Geometry check sheet. Reference: the model listing, model coordinates, mm. Face numbers are marked on the shaded views. Round coordinates to 2 decimals unless told otherwise and drop trailing zeros. Write each loop counter-clockwise with the first axis right and the second up, starting at its lowest first coordinate (ties: lowest second). Pieces come first, ordered by that corner, then holes. Notation, with made-up numbers: (-0.5, -22.5) - (47.5, -22.5) arc R18 ccw to (47.5, -11.5) - close; hole circle Ø11 at (6, 49.5). An arc over 180 degrees is marked (long way). Return JSON: item names as keys, results as strings. Group by question number.
from build123d import *

# Parameters (mm, degrees)
SKETCH2_R           = 21
BOSS_EXTRUDE1_DEPTH = 10
CUT_EXTRUDE1_REACH  = 77.44
SKETCH3_R           = 1.75
SKETCH5_W           = 4
SKETCH5_H           = 1


with BuildPart() as part:
    # Sketch2 → Boss-Extrude1 (new body)
    # profile 1 of 6: a face of its own
    with BuildSketch(Plane(origin=(0, 0, 0), x_dir=(1, 0, 0), z_dir=(0, 1, 0))):
        with BuildLine():
            ThreePointArc((-39.742001703, 30.095205518), (-35.527778851, 29.794741171), (-31.819805153, 31.819805153))
            Line((-31.819805153, 31.819805153), (-42.426406871, 42.426406871))
            ThreePointArc((-42.426406871, 42.426406871), (-44.451470854, 35.527778851), (-39.742001703, 30.095205518))
        make_face()
    # profile 2 of 6: a face of its own
    with BuildSketch(Plane(origin=(0, 0, 0), x_dir=(1, 0, 0), z_dir=(0, 1, 0))):
        with BuildLine():
            Line((-42.426406871, 42.426406871), (-31.819805153, 31.819805153))
            ThreePointArc((-31.819805153, 31.819805153), (0, 45), (31.819805153, 31.819805153))
            ThreePointArc((31.819805153, 31.819805153), (35.527778851, 29.794741171), (39.742001703, 30.095205518))
            ThreePointArc((39.742001703, 30.095205518), (44.451470854, 35.527778851), (42.426406871, 42.426406871))
            ThreePointArc((42.426406871, 42.426406871), (0, 60), (-42.426406871, 42.426406871))
        make_face()
    # profile 3 of 6: a face of its own
    with BuildSketch(Plane(origin=(0, 0, 0), x_dir=(1, 0, 0), z_dir=(0, 1, 0))):
        with BuildLine():
            ThreePointArc((31.819805153, 31.819805153), (0, 45), (-31.819805153, 31.819805153))
            ThreePointArc((-31.819805153, 31.819805153), (-33.665365801, 29.860394262), (-35.390472848, 27.794143836))
            add(Edge.make_bspline(
                [(-35.390472848, 27.794143836), (-32.245912853, 25.570807212), (-24.806129807, 15.839794796), (-24.750821328, 4.074395815), (-23.058627279, -4.533178579)],
                knots=[0.115209689, 0.115209689, 0.115209689, 0.115209689, 0.392292763, 1, 1, 1, 1], degree=3))
            ThreePointArc((-23.058627279, -4.533178579), (-2.277307506, 23.38939654), (23.5, 0))
            ThreePointArc((23.5, 0), (23.38939654, -2.277307506), (23.058627279, -4.533178579))
            add(Edge.make_bspline(
                [(35.390472848, 27.794143836), (32.245912853, 25.570807212), (24.806129807, 15.839794796), (24.750821328, 4.074395815), (23.058627279, -4.533178579)],
                knots=[0.115209689, 0.115209689, 0.115209689, 0.115209689, 0.392292763, 1, 1, 1, 1], degree=3))
            ThreePointArc((35.390472848, 27.794143836), (33.665365801, 29.860394262), (31.819805153, 31.819805153))
        make_face()
    # profile 4 of 6: a face of its own
    with BuildSketch(Plane(origin=(0, 0, 0), x_dir=(1, 0, 0), z_dir=(0, 1, 0))):
        with BuildLine():
            ThreePointArc((-35.390472848, 27.794143836), (-33.665365801, 29.860394262), (-31.819805153, 31.819805153))
            ThreePointArc((-31.819805153, 31.819805153), (-35.527778851, 29.794741171), (-39.742001703, 30.095205518))
            add(Edge.make_bspline(
                [(-39.742001703, 30.095205518), (-38.146305527, 29.500581015), (-36.697964408, 28.718595549), (-35.390472848, 27.794143836)],
                knots=[0, 0, 0, 0, 0.115209689, 0.115209689, 0.115209689, 0.115209689], degree=3))
        make_face()
    # profile 5 of 6: a face of its own
    with BuildSketch(Plane(origin=(0, 0, 0), x_dir=(1, 0, 0), z_dir=(0, 1, 0))):
        with BuildLine():
            ThreePointArc((39.742001703, 30.095205518), (35.527778851, 29.794741171), (31.819805153, 31.819805153))
            ThreePointArc((31.819805153, 31.819805153), (33.665365801, 29.860394262), (35.390472848, 27.794143836))
            add(Edge.make_bspline(
                [(39.742001703, 30.095205518), (38.146305527, 29.500581015), (36.697964408, 28.718595549), (35.390472848, 27.794143836)],
                knots=[0, 0, 0, 0, 0.115209689, 0.115209689, 0.115209689, 0.115209689], degree=3))
        make_face()
    # profile 6 of 6: a face of its own
    with BuildSketch(Plane(origin=(0, 0, 0), x_dir=(1, 0, 0), z_dir=(0, 1, 0))):
        with BuildLine():
            ThreePointArc((23.5, 0), (-2.277307506, 23.38939654), (-23.058627279, -4.533178579))
            ThreePointArc((-23.058627279, -4.533178579), (0, -23.5), (23.058627279, -4.533178579))
            ThreePointArc((23.058627279, -4.533178579), (23.38939654, -2.277307506), (23.5, 0))
        make_face()
        with Locations(Location((0, 0, 0), (0, 0, 270))):
            Circle(SKETCH2_R, mode=Mode.SUBTRACT)
    extrude(amount=BOSS_EXTRUDE1_DEPTH)

    # Sketch3 → Cut-Extrude1 (cut, up to next)
    with BuildSketch(Plane(origin=(0, 10, 0), x_dir=(1, 0, 0), z_dir=(0, 1, 0)), mode=Mode.PRIVATE) as cut_extrude1_sk1:
        with Locations(Location((-37.123106012, 37.123106012, 0), (0, 0, 270))):
            Circle(SKETCH3_R)
    cut_extrude1_tool1 = extrude(cut_extrude1_sk1.sketch, amount=-CUT_EXTRUDE1_REACH, mode=Mode.PRIVATE) & part.part
    # Sketch3 → Cut-Extrude1 (cut, up to next)
    with BuildSketch(Plane(origin=(0, 10, 0), x_dir=(1, 0, 0), z_dir=(0, 1, 0)), mode=Mode.PRIVATE) as cut_extrude1_sk2:
        with Locations(Location((37.123106012, 37.123106012, 0), (0, 0, 270))):
            Circle(SKETCH3_R)
    cut_extrude1_tool2 = extrude(cut_extrude1_sk2.sketch, amount=-CUT_EXTRUDE1_REACH, mode=Mode.PRIVATE) & part.part
    add(cut_extrude1_tool1.solids().sort_by_distance((-37.123106, 10, -37.123106))[0], mode=Mode.SUBTRACT)
    add(cut_extrude1_tool2.solids().sort_by_distance((37.123106, 10, -37.123106))[0], mode=Mode.SUBTRACT)

    # Sketch5 → Revolve1 (revolve)
    with BuildSketch(Plane.XY, mode=Mode.PRIVATE) as revolve1_sk:
        with Locations((-21.058627279, 7.5)):
            Rectangle(SKETCH5_W, SKETCH5_H)
    revolve(revolve1_sk.sketch.rotate(Axis((0, 10, 0), (0, -1, 0)), 270), axis=Axis((0, 10, 0), (0, -1, 0)))


solid = part.part
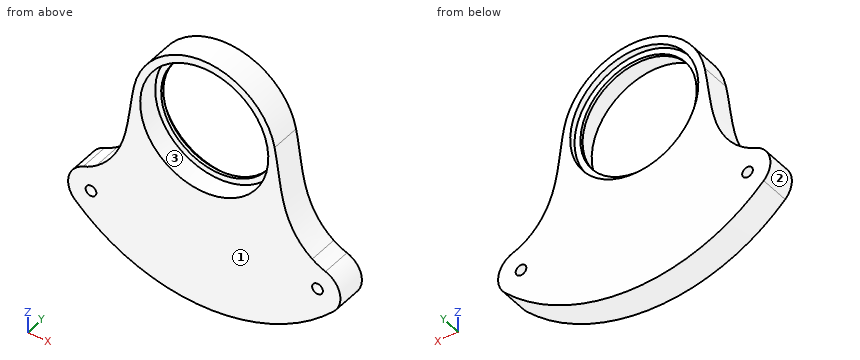
1. Material ranges on line 1 along X through (y, z) = (1.75, -38); line 2 along Z through (x, y) = (0, 9.5); line 3 along Z through (x, y) = (11, 1.75), recorded low to high.
2. Mould release check, pull along Z, two halves, no side actions. Record for the marked faces 1, 2 and 3: pulls with the +Z half, pulls with the -Z half, needs draft (parallel to the pull), parting line crosses it, or undercut.
3. Section check A-A (z = 12.5). Enter the section's corners in (x, y), and give its area (3 significant figures).
4. Section check C-C (y = 6). State how many separate pieces and enclosed holes the cut face has, and give its area (3 significant figures).
5. Section check B-B (x = 5.5). Enter the section's corners in (y, z), and give its area (3 significant figures).
6. Depth check by flat-ended pin: pin 1 Ø2 at (y, z) = (8.5, -32.5) entering from +X; pin 2 Ø6 at (y, z) = (4.5, -48) entering from -X; pin 3 Ø2 at (x, y) = (17, 5.5) entering from -Z. Enter the tip coordinate at first touch or a pass-through.
Result sheet:
{
 "1": {"line 1": "x = -44.57 to -38.64, -35.61 to 35.61, 38.64 to 44.57", "line 2": "z = -60 to -21, 21 to 23.5", "line 3": "z = -58.98 to -17.89, 17.89 to 20.77"},
 "2": {"face 1": "needs draft", "face 2": "parting line crosses it", "face 3": "undercut"},
 "3": {"outline": "(-19.9, 0) - (-16.87, 0) - (-16.87, 7) - (-14.39, 7) - (-14.39, 8) - (-16.87, 8) - (-16.87, 10) - (-19.9, 10) - close; (14.39, 7) - (16.87, 7) - (16.87, 0) - (19.9, 0) - (19.9, 10) - (16.87, 10) - (16.87, 8) - (14.39, 8) - close", "area": "65.5 mm²"},
 "4": {"separate pieces": "1", "enclosed holes": "3", "area": "3,250 mm²"},
 "5": {"outline": "(0, -59.75) - (10, -59.75) - (10, -20.27) - (8, -20.27) - (8, -18.25) - (7, -18.25) - (7, -20.27) - (0, -20.27) - close; (0, 20.27) - (7, 20.27) - (7, 18.25) - (8, 18.25) - (8, 20.27) - (10, 20.27) - (10, 22.85) - (0, 22.85) - close", "area": "425 mm²"},
 "6": {"pin 1": "stops at x = 43.69", "pin 2": "stops at x = -39.69", "pin 3": "stops at z = -57.83"}
}
